CAD build for the part. Positions are in the model's coordinates, mm. A direction names the side the tool comes from. Round coordinates to 2 decimals unless told otherwise and drop trailing zeros. Loops run counter-clockwise (first coordinate to the right, second up) from the corner with the lowest first, then second, coordinate; pieces in that order, holes last. Notation, with made-up numbers: (15, 59.5) - (44, 59.5) arc R19 cw to (44, 65.5) - close; hole circle Ø3 at (46, 79.5). An arc over 180 degrees is marked (long way). One line per question, with ' | ' between items.
```python
from build123d import *

# Parameters (mm, degrees)
ESQUISSE1_W                          = 114.45
ESQUISSE1_H                          = 65.45
BOSS_EXTRU_1_DEPTH                   = 1.6
BOSS_EXTRU_2_DEPTH                   = 14
ESQUISSE3_R                          = 3.9
BOSS_EXTRU_3_DEPTH                   = 5.8
ESQUISSE6_W                          = 10
ESQUISSE6_H                          = 18.25
BOSS_EXTRU_6_DEPTH                   = 15.5
R_P_TITION_LIN_AIRE1_COUNT           = 2
R_P_TITION_LIN_AIRE1_PITCH           = 28.1
R_P_TITION_LIN_AIRE2_COUNT           = 2
R_P_TITION_LIN_AIRE2_PITCH           = 57.15
R_P_TITION_LIN_AIRE2_COPY_1_DEPTH    = 14
R_P_TITION_LIN_AIRE2_COPY_2_SKETCH_R = 3.9
R_P_TITION_LIN_AIRE2_COPY_2_DEPTH    = 5.8
R_P_TITION_LIN_AIRE2_COPY_3_SKETCH_W = 10
R_P_TITION_LIN_AIRE2_COPY_3_SKETCH_H = 18.25
R_P_TITION_LIN_AIRE2_COPY_3_DEPTH    = 15.5
BOSS_EXTRU_4_DEPTH                   = 14
ESQUISSE5_R                          = 3.9
BOSS_EXTRU_5_DEPTH                   = 5.6
CONG_1_R                             = 3
ESQUISSE7_W                          = 54
ESQUISSE7_H                          = 25.5
BOSS_EXTRU_7_DEPTH                   = 16.4


with BuildPart() as part:
    # Esquisse1 → Boss.-Extru.1 (new body)
    with BuildSketch(Plane(origin=(0, 0, 0), x_dir=(1, 0, 0), z_dir=(0, 1, 0))):
        Rectangle(ESQUISSE1_W, ESQUISSE1_H)
    extrude(amount=BOSS_EXTRU_1_DEPTH)

    # Esquisse2 → Boss.-Extru.2 (add)
    with BuildSketch(Plane.XY.offset(32.725)):
        with BuildLine():
            Line((44.525, 1.6), (55.325, 1.6))
            Line((55.325, 1.6), (55.325, 7.9))
            ThreePointArc((55.325, 7.9), (49.925, 13.3), (44.525, 7.9))
            Line((44.525, 7.9), (44.525, 1.6))
        make_face()
    boss_extru_2 = extrude(amount=-BOSS_EXTRU_2_DEPTH)

    # Esquisse3 → Boss.-Extru.3 (add)
    with BuildSketch(Plane.XY.offset(32.725)):
        with Locations((49.925, 7.9)):
            Circle(ESQUISSE3_R)
    boss_extru_3 = extrude(amount=BOSS_EXTRU_3_DEPTH)

    # Esquisse6 → Boss.-Extru.6 (add)
    with BuildSketch(Plane(origin=(0, 1.6, 0), x_dir=(1, 0, 0), z_dir=(0, 1, 0))):
        with Locations((36.925, -8.4)):
            Rectangle(ESQUISSE6_W, ESQUISSE6_H)
    boss_extru_6 = extrude(amount=BOSS_EXTRU_6_DEPTH)

    # Répétition linéaire1: Boss.-Extru.2, Boss.-Extru.3, Boss.-Extru.6 ×2
    with Locations(*[(-i * R_P_TITION_LIN_AIRE1_PITCH, 0, 0) for i in range(1, R_P_TITION_LIN_AIRE1_COUNT)]):
        add(boss_extru_2)
        add(boss_extru_3)
        add(boss_extru_6)

    # Répétition linéaire2: Boss.-Extru.2, Boss.-Extru.3, Boss.-Extru.6 ×2
    with Locations(*[(-i * R_P_TITION_LIN_AIRE2_PITCH, 0, 0) for i in range(1, R_P_TITION_LIN_AIRE2_COUNT)]):
        add(boss_extru_2)
        add(boss_extru_3)
        add(boss_extru_6)

    # Répétition linéaire2 copy 1 sketch → Répétition linéaire2 copy 1 (add)
    with BuildSketch(Plane(origin=(-85.25, 0, 32.725), x_dir=(1, 0, 0), z_dir=(0, 0, 1))):
        with BuildLine():
            Line((44.525, 1.6), (55.325, 1.6))
            Line((55.325, 1.6), (55.325, 7.9))
            ThreePointArc((55.325, 7.9), (49.925, 13.3), (44.525, 7.9))
            Line((44.525, 7.9), (44.525, 1.6))
        make_face()
    extrude(amount=-R_P_TITION_LIN_AIRE2_COPY_1_DEPTH)

    # Répétition linéaire2 copy 2 sketch → Répétition linéaire2 copy 2 (add)
    with BuildSketch(Plane(origin=(-85.25, 0, 32.725), x_dir=(1, 0, 0), z_dir=(0, 0, 1))):
        with Locations((49.925, 7.9)):
            Circle(R_P_TITION_LIN_AIRE2_COPY_2_SKETCH_R)
    extrude(amount=R_P_TITION_LIN_AIRE2_COPY_2_DEPTH)

    # Répétition linéaire2 copy 3 sketch → Répétition linéaire2 copy 3 (add)
    with BuildSketch(Plane(origin=(-85.25, 1.6, 0), x_dir=(1, 0, 0), z_dir=(0, 1, 0))):
        with Locations((36.925, -8.4)):
            Rectangle(R_P_TITION_LIN_AIRE2_COPY_3_SKETCH_W, R_P_TITION_LIN_AIRE2_COPY_3_SKETCH_H)
    extrude(amount=R_P_TITION_LIN_AIRE2_COPY_3_DEPTH)

    # Esquisse4 → Boss.-Extru.4 (add)
    with BuildSketch(Plane(origin=(0, 0, -32.725), x_dir=(-1, 0, 0), z_dir=(0, 0, -1))):
        with BuildLine():
            Line((-41.675, 1.6), (-52.475, 1.6))
            Line((-52.475, 1.6), (-52.475, 7.9))
            ThreePointArc((-52.475, 7.9), (-47.075, 13.3), (-41.675, 7.9))
            Line((-41.675, 7.9), (-41.675, 1.6))
        make_face()
    extrude(amount=-BOSS_EXTRU_4_DEPTH)

    # Esquisse5 → Boss.-Extru.5 (add)
    with BuildSketch(Plane(origin=(0, 0, -32.725), x_dir=(-1, 0, 0), z_dir=(0, 0, -1))):
        with Locations((-47.075, 7.9)):
            Circle(ESQUISSE5_R)
    extrude(amount=BOSS_EXTRU_5_DEPTH)

    # Congé1
    cong_1_edges = [part.edges().sort_by_distance(p)[0] for p in [
        (57.225, 0.8, -32.725),
        (-57.225, 0.8, -32.725),
        (-57.225, 0.8, 32.725),
        (57.225, 0.8, 32.725),
    ]]
    fillet(cong_1_edges, radius=CONG_1_R)

    # Esquisse7 → Boss.-Extru.7 (add)
    with BuildSketch(Plane(origin=(0, 1.6, 0), x_dir=(1, 0, 0), z_dir=(0, 1, 0))):
        with Locations((-26.725, 17.975)):
            Rectangle(ESQUISSE7_W, ESQUISSE7_H)
    extrude(amount=BOSS_EXTRU_7_DEPTH)


solid = part.part
```
(1) Probe L1, parallel to X at y = 4.25, z = 28 (3 decimals); L2, parallel to X at y = 16, z = 0 (3 decimals); L3, parallel to Z at x = -23.5, y = 15.5 (3 decimals). List the from-to ranges inside material, lowest first.
Results found:
L1: x = -40.725 to -29.925, -12.625 to -1.825, 16.425 to 27.225, 44.525 to 55.325 | L2: x = -53.325 to -43.325, -25.225 to -15.225, 3.825 to 13.825, 31.925 to 41.925 | L3: z = -30.725 to -5.225, -0.725 to 17.525
(2) Two-plate mould, pull along X, no slides. Class faces 5 (the face through (-53.725, 10, -18)), 6 (the face through (50, 8, 18.725)), 7 (the face through (16.425, 5, 26)): released by +X, released by -X, zero draft, split by the parting line, or undercut.
Results found:
face 5: released by -X | face 6: zero draft | face 7: undercut
(3) Cut at D-D, the plane y = 6.25. State how many separate pieces and enclosed holes the cut face has, then the cut area to 3 significant figures.
Results found:
separate pieces: 10 | enclosed holes: 0 | area: 3,070 mm²
(4) Tool access for faces 1 (the face through (52.475, 5, -26)), 2 (the face through (-48, 9, -0.725)), 3 (the face through (37, 9, 17.525)), 4 (the face through (-3.505, 9.071, 35.584)): list every direction of +Z, -Z, +X, -X, +Y, -Y with a clear straight run to the whole face (end or side of a thin tool).
Results found:
face 1: -Z, +X, +Y | face 2: +X, -X, +Y | face 3: +Z, +X, -X, +Y | face 4: +Z
(5) Cut at B-B, the plane x = 39. Write the cut outline in (y, z) (3 decimals).
Results found:
outline: (0, -32.725) - (1.6, -32.725) - (1.6, -0.725) - (17.1, -0.725) - (17.1, 17.525) - (1.6, 17.525) - (1.6, 32.725) - (0, 32.725) - close
(6) Cut at C-C, the plane z = -14. Write the cut outline in (x, y) (3 decimals), then the cut area to 3 significant figures.
Results found:
outline: (-57.225, 0) - (57.225, 0) - (57.225, 1.6) - (0.275, 1.6) - (0.275, 18) - (-53.725, 18) - (-53.725, 1.6) - (-57.225, 1.6) - close | area: 1,070 mm²
(7) Cut at A-A, the plane y = 14.5. Write the cut outline in (x, z) (3 decimals).
Results found:
outline: (-53.725, -30.725) - (0.275, -30.725) - (0.275, -5.225) - (-53.725, -5.225) - close; (-53.325, -0.725) - (-43.325, -0.725) - (-43.325, 17.525) - (-53.325, 17.525) - close; (-25.225, -0.725) - (-15.225, -0.725) - (-15.225, 17.525) - (-25.225, 17.525) - close; (3.825, -0.725) - (13.825, -0.725) - (13.825, 17.525) - (3.825, 17.525) - close; (31.925, -0.725) - (41.925, -0.725) - (41.925, 17.525) - (31.925, 17.525) - close
(8) Drop flat-ended pins along their axis: P1, Ø5.5, axis at x = -36.5, y = 7, coming from the -Z side (3 decimals); P2, Ø10, axis at x = -25.5, z = 19.5, coming from the +Y side; P3, Ø7, axis at y = 6, z = 27, coming from the +X side (3 decimals). Give the stop position or say it passes through.
Results found:
P1: stops at z = -30.725 | P2: stops at y = 17.1 | P3: stops at x = 55.325
